Check sheet for the modelled part. Datum: model origin and axes. Units: mm. Coordinates: 2 decimals unless noted, no trailing zeros.
```python
from build123d import *

# Parameters (mm, degrees)
SKETCH1_W             = 130
SKETCH1_H             = 70
SKETCH1_R             = 1.725
SKETCH1_R_2           = 1.13
SKETCH1_R_3           = 0.8
SKETCH1_R_4           = 1.5
BOSS_EXTRUDE1_DEPTH   = 6.35
F_4_40_TAPPED_HOLE1_D = 2.2606
FILLET1_R             = 1


with BuildPart() as part:
    # Sketch1 → Boss-Extrude1 (new body)
    with BuildSketch(Plane(origin=(0, 0, 0), x_dir=(1, 0, 0), z_dir=(0, 1, 0))):
        with Locations((65, -35)):
            Rectangle(SKETCH1_W, SKETCH1_H)
        with Locations((10, -10)):
            Circle(SKETCH1_R, mode=Mode.SUBTRACT)
        with Locations((20, -10)):
            Circle(SKETCH1_R_2, mode=Mode.SUBTRACT)
        with Locations((30, -10)):
            Circle(SKETCH1_R_2, mode=Mode.SUBTRACT)
        with Locations((40, -10)):
            Circle(SKETCH1_R_2, mode=Mode.SUBTRACT)
        with Locations((45, -17.5)):
            Circle(SKETCH1_R_2, mode=Mode.SUBTRACT)
        with Locations((40, -17.5)):
            Circle(SKETCH1_R, mode=Mode.SUBTRACT)
        with Locations((27, -27)):
            Circle(SKETCH1_R_3, mode=Mode.SUBTRACT)
        with Locations((27, -19.6)):
            Circle(SKETCH1_R_4, mode=Mode.SUBTRACT)
        with Locations((27, -43)):
            Circle(SKETCH1_R_3, mode=Mode.SUBTRACT)
        with Locations((27, -50.4)):
            Circle(SKETCH1_R_4, mode=Mode.SUBTRACT)
        with Locations((45, -52.5)):
            Circle(SKETCH1_R_2, mode=Mode.SUBTRACT)
        with Locations((40, -52.5)):
            Circle(SKETCH1_R, mode=Mode.SUBTRACT)
        with Locations((40, -60)):
            Circle(SKETCH1_R_2, mode=Mode.SUBTRACT)
        with Locations((30, -60)):
            Circle(SKETCH1_R_2, mode=Mode.SUBTRACT)
        with Locations((20, -60)):
            Circle(SKETCH1_R_2, mode=Mode.SUBTRACT)
        with Locations((10, -60)):
            Circle(SKETCH1_R, mode=Mode.SUBTRACT)
        with Locations((120, -60)):
            Circle(SKETCH1_R, mode=Mode.SUBTRACT)
        with Locations((110, -60)):
            Circle(SKETCH1_R_2, mode=Mode.SUBTRACT)
        with Locations((100, -60)):
            Circle(SKETCH1_R_2, mode=Mode.SUBTRACT)
        with Locations((90, -60)):
            Circle(SKETCH1_R_2, mode=Mode.SUBTRACT)
        with Locations((85, -52.5)):
            Circle(SKETCH1_R_2, mode=Mode.SUBTRACT)
        with Locations((90, -52.5)):
            Circle(SKETCH1_R, mode=Mode.SUBTRACT)
        with Locations((103, -43)):
            Circle(SKETCH1_R_3, mode=Mode.SUBTRACT)
        with Locations((103, -50.4)):
            Circle(SKETCH1_R_4, mode=Mode.SUBTRACT)
        with Locations((103, -19.6)):
            Circle(SKETCH1_R_4, mode=Mode.SUBTRACT)
        with Locations((103, -27)):
            Circle(SKETCH1_R_3, mode=Mode.SUBTRACT)
        with Locations((85, -17.5)):
            Circle(SKETCH1_R_2, mode=Mode.SUBTRACT)
        with Locations((90, -17.5)):
            Circle(SKETCH1_R, mode=Mode.SUBTRACT)
        with Locations((90, -10)):
            Circle(SKETCH1_R_2, mode=Mode.SUBTRACT)
        with Locations((100, -10)):
            Circle(SKETCH1_R_2, mode=Mode.SUBTRACT)
        with Locations((110, -10)):
            Circle(SKETCH1_R_2, mode=Mode.SUBTRACT)
        with Locations((120, -10)):
            Circle(SKETCH1_R, mode=Mode.SUBTRACT)
    extrude(amount=BOSS_EXTRUDE1_DEPTH)

    # #4-40 Tapped Hole1 (through all)
    with Locations(Plane(origin=(40, 6.35, 10), x_dir=(0, 0, 1), z_dir=(0, 1, 0))):
        with Locations((0, 0), (0, -10), (0, -20), (0, 50), (50, 70), (50, 60), (50, 50), (50, 0), (50, -10), (50, -20), (0, 70), (0, 60), (7.5, 5), (7.5, 45), (42.5, 45), (42.5, 5)):
            Hole(F_4_40_TAPPED_HOLE1_D / 2)

    # Fillet1
    fillet1_edges = [part.edges().sort_by_distance(p)[0] for p in [
        (130, 3.175, 70),
        (0, 3.175, 70),
        (0, 3.175, 0),
        (130, 3.175, 0),
    ]]
    fillet(fillet1_edges, radius=FILLET1_R)


solid = part.part
```
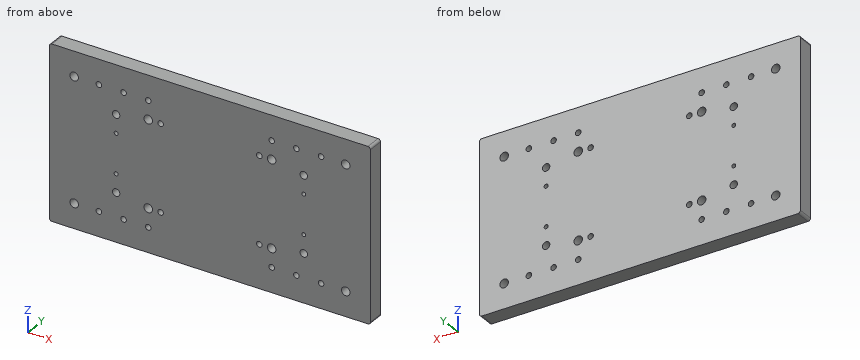
1) Section check A-A on y = 4.25. Give the number of separate pieces and of enclosed holes in the cut face, plus the area to 3 significant figures.
Answer sheet:
separate pieces: 1
enclosed holes: 32
area: 8,920 mm2
2) Scan lines: line 1 (Z direction, x = 110, y = 3.75); line 2 (Z direction, x = 103, y = 4); line 3 (X direction, y = 1.5, z = 50.4). Record each from-to range of solid material in increasing order.
Answer sheet:
line 1: z = 0 to 8.87, 11.13 to 58.87, 61.13 to 70
line 2: z = 0 to 18.1, 21.1 to 26.2, 27.8 to 42.2, 43.8 to 48.9, 51.9 to 70
line 3: x = 0 to 25.5, 28.5 to 101.5, 104.5 to 130
3) Depth check by flat-ended pin: pin 1 (1.8 mm diameter, centred on x = 27, z = 43, fed in from +Y); pin 2 (2 mm diameter, centred on x = 10, z = 10, fed in from +Y). Enter the tip coordinate at first touch or a pass-through.
Answer sheet:
pin 1: stops at y = 6.35
pin 2: passes through
